Verification items for the finished model (mm, model axes). A direction names the side the tool comes from. Round coordinates to 2 decimals unless told otherwise and drop trailing zeros. Write each loop counter-clockwise with the first axis right and the second up, starting at its lowest first coordinate (ties: lowest second). Pieces come first, ordered by that corner, then holes. Notation, with made-up numbers: M 39,-28 L 59,-28 A24 ccw 59,-1 Z; hole C -4,32 d9. An arc over 180 degrees is marked long. One line per question, with ' | ' between items. Start each with the question number.
Q1. Cross-section at D-D (x = -20). Record the boundary of the cut face in (y, z), then the cut area to 3 significant figures.
Q2. Cross-section at B-B (x = 8.5). Record the boundary of the cut face in (y, z).
Q3. Gauge pin test, flat ends, axial feed: pin 1 (2 mm diameter, centred on y = 11.5, z = -5, fed in from +X); pin 2 (4.5 mm diameter, centred on x = -54, y = 12.5, fed in from -Z); pin 3 (2 mm diameter, centred on x = -54.5, y = -1, fed in from +Z). Record the tip position at first contact, or that the pin passes through.
Q4. Release check for a two-part mould opening along X. For faces 1 (the face through (-55, -2.7, -3)), 2 (the face through (-55, -3, -10)), 3 (the face through (-65, 25, 2)) record: released by +X, released by -X, zero draft, split by the parting line, or undercut.
Q5. Thickness scan on line 1 along Y through (x, z) = (30, 11.2); line 2 along Y through (x, z) = (30, 2.4); line 3 along X through (y, z) = (-4.45, -5). Record the ranges inside material, lowest first. Write a range as from..to.
Q6. Tool access check on faces 4 (the face through (-63, 12, -4)), 5 (the face through (23, -3, -5)), 6 (the face through (15, 10.2, -3)). Record the directions out of +Z, -Z, +X, -X, +Y, -Y that give a thin tool (end or side, any length) a straight path to the whole face; none if there is none.
Q7. Cross-section at A-A (x = 30). Record the boundary of the cut face in (y, z), then the cut area to 3 significant figures.
Q8. Cross-section at C-C (y = 116). Record the boundary of the cut face in (x, z).
from build123d import *

# Parameters (mm, degrees)
EXTRUDE_START                = 0.2
EXTRUDE_312_DEPTH            = 4
CUT_EXTRUDE_453_DEPTH        = 142.840191765
CUT_EXTRUDE_453_DEPTH_BACK   = 142.840191765
EXTRUDE_START_2              = -8
SKETCH_3_W                   = 16
SKETCH_3_H                   = 4
EXTRUDE_645_DEPTH            = 12.2
EXTRUDE_START_3              = -10
SKETCH_4_W                   = 16
SKETCH_4_H                   = 2.7
EXTRUDE_849_DEPTH            = 14.2
EXTRUDE_START_4              = -2.7
SKETCH_5_W                   = 16
SKETCH_5_H                   = 14.2
SKETCH_5_W_2                 = 6.7
SKETCH_5_H_2                 = 5.8
EXTRUDE_M3_DEPTH             = 2.5
SKETCH_6_W                   = 6
SKETCH_6_H                   = 45
EXTRUDE_1326_DEPTH           = 12.6
EXTRUDE_START_5              = 8.8
SKETCH_7_W                   = 50
SKETCH_7_H                   = 45
EXTRUDE_1474_DEPTH           = 4
CUT_EXTRUDE_3P4_DEPTH        = 143.354627603
CUT_EXTRUDE_3P4_DEPTH_BACK   = 143.354627603
SKETCH_8_R                   = 1.7
CUT_EXTRUDE_3P4_2_DEPTH      = 143.354627603
CUT_EXTRUDE_3P4_2_DEPTH_BACK = 143.354627603
SKETCH_9_R                   = 1.7


with BuildPart() as part:
    # 草图1 → Extrude 312 (new body)
    with BuildSketch(Plane.XY.offset(EXTRUDE_START)):
        Polygon((-65, -5.4), (40, -5.4), (40, 126), (-10, 126), (-65, 55), align=None)
    extrude(amount=EXTRUDE_312_DEPTH)

    # 草图2 → Cut-Extrude 453 (cut, two sides: drawn at the far end of the back side and taken through both)
    with BuildSketch(Plane.XY.offset(-CUT_EXTRUDE_453_DEPTH_BACK)):
        Polygon((-55, 15.2), (20, 15.2), (20, 105), (-4, 105), (-55, 49), align=None)
    extrude(amount=CUT_EXTRUDE_453_DEPTH + CUT_EXTRUDE_453_DEPTH_BACK, mode=Mode.SUBTRACT)

    # 草图3 → Extrude 645 (add)
    with BuildSketch(Plane.XY.offset(EXTRUDE_START_2)):
        with Locations((-55, 12.2)):
            Rectangle(SKETCH_3_W, SKETCH_3_H)
        with Locations((15, 12.2)):
            Rectangle(SKETCH_3_W, SKETCH_3_H)
    extrude(amount=EXTRUDE_645_DEPTH)

    # 草图4 → Extrude 849 (add)
    with BuildSketch(Plane.XY.offset(EXTRUDE_START_3)):
        with Locations((-55, -4.05)):
            Rectangle(SKETCH_4_W, SKETCH_4_H)
        with Locations((15, -4.05)):
            Rectangle(SKETCH_4_W, SKETCH_4_H)
    extrude(amount=EXTRUDE_849_DEPTH)

    # 草图5 → 下卡唇M3螺母防转槽 (add)
    # profile 1 of 2: a face of its own
    with BuildSketch(Plane(origin=(0, 0, 0), x_dir=(1, 0, 0), z_dir=(0, 1, 0)).offset(EXTRUDE_START_4)):
        with Locations((-55, 2.9)):
            Rectangle(SKETCH_5_W, SKETCH_5_H)
        with Locations((-55, 5)):
            Rectangle(SKETCH_5_W_2, SKETCH_5_H_2, mode=Mode.SUBTRACT)
    # profile 2 of 2: a face of its own
    with BuildSketch(Plane(origin=(0, 0, 0), x_dir=(1, 0, 0), z_dir=(0, 1, 0)).offset(EXTRUDE_START_4)):
        with Locations((15, 2.9)):
            Rectangle(SKETCH_5_W, SKETCH_5_H)
        with Locations((15, 5)):
            Rectangle(SKETCH_5_W_2, SKETCH_5_H_2, mode=Mode.SUBTRACT)
    extrude(amount=EXTRUDE_M3_DEPTH)

    # 草图6 → Extrude 1326 (add)
    with BuildSketch(Plane.XY.offset(EXTRUDE_START)):
        with Locations((-7, 103.5)):
            Rectangle(SKETCH_6_W, SKETCH_6_H)
    extrude(amount=EXTRUDE_1326_DEPTH)

    # 草图7 → Extrude 1474 (add)
    with BuildSketch(Plane.XY.offset(EXTRUDE_START_5)):
        with Locations((15, 103.5)):
            Rectangle(SKETCH_7_W, SKETCH_7_H)
    extrude(amount=EXTRUDE_1474_DEPTH)

    # 草图8 → Cut-Extrude 3p4 (cut, two sides: drawn at the far end of the back side and taken through both)
    with BuildSketch(Plane.XY.offset(-CUT_EXTRUDE_3P4_DEPTH_BACK)):
        with Locations((30, 91)):
            Circle(SKETCH_8_R)
        with Locations((30, 116)):
            Circle(SKETCH_8_R)
    extrude(amount=CUT_EXTRUDE_3P4_DEPTH + CUT_EXTRUDE_3P4_DEPTH_BACK, mode=Mode.SUBTRACT)

    # 草图9 → Cut-Extrude 3p4 2 (cut, two sides: drawn at the far end of the back side and taken through both)
    with BuildSketch(Plane(origin=(0, 0, 0), x_dir=(1, 0, 0), z_dir=(0, 1, 0)).offset(-CUT_EXTRUDE_3P4_2_DEPTH_BACK)):
        with Locations(Location((-55, 5, 0), (0, 0, 270))):
            Circle(SKETCH_9_R)
        with Locations(Location((15, 5, 0), (0, 0, 270))):
            Circle(SKETCH_9_R)
    extrude(amount=CUT_EXTRUDE_3P4_2_DEPTH + CUT_EXTRUDE_3P4_2_DEPTH_BACK, mode=Mode.SUBTRACT)


solid = part.part
Determined:
1) outline: M -5.4,0.2 L 15.2,0.2 L 15.2,4.2 L -5.4,4.2 Z; M 87.43,0.2 L 113.09,0.2 L 113.09,4.2 L 87.43,4.2 Z | area: 185 mm²
2) outline: M -5.4,-10 L -0.2,-10 L -0.2,0.2 L 10.2,0.2 L 10.2,-8 L 14.2,-8 L 14.2,0.2 L 15.2,0.2 L 15.2,4.2 L -5.4,4.2 Z; M 81,8.8 L 126,8.8 L 126,12.8 L 81,12.8 Z; M 105,0.2 L 126,0.2 L 126,4.2 L 105,4.2 Z
3) pin 1: stops at x = 23 | pin 2: stops at z = -8 | pin 3: stops at z = 4.2
4) face 1: undercut | face 2: zero draft | face 3: released by -X
5) line 1: y = 81..89.3, 92.7..114.3, 117.7..126 | line 2: y = -5.4..89.3, 92.7..114.3, 117.7..126 | line 3: x = -63..-56.7, -53.3..-47, 7..13.3, 16.7..23
6) face 4: -Z, -X, +Y, -Y | face 5: -Z, +X, +Y, -Y | face 6: -Z, +X, -X
7) outline: M -5.4,0.2 L 89.3,0.2 L 89.3,4.2 L -5.4,4.2 Z; M 81,8.8 L 89.3,8.8 L 89.3,12.8 L 81,12.8 Z; M 92.7,0.2 L 114.3,0.2 L 114.3,4.2 L 92.7,4.2 Z; M 92.7,8.8 L 114.3,8.8 L 114.3,12.8 L 92.7,12.8 Z; M 117.7,0.2 L 126,0.2 L 126,4.2 L 117.7,4.2 Z; M 117.7,8.8 L 126,8.8 L 126,12.8 L 117.7,12.8 Z | area: 651 mm²
8) outline: M -17.75,0.2 L 28.3,0.2 L 28.3,4.2 L -4,4.2 L -4,8.8 L 28.3,8.8 L 28.3,12.8 L -10,12.8 L -10,4.2 L -17.75,4.2 Z; M 31.7,0.2 L 40,0.2 L 40,4.2 L 31.7,4.2 Z; M 31.7,8.8 L 40,8.8 L 40,12.8 L 31.7,12.8 Z
